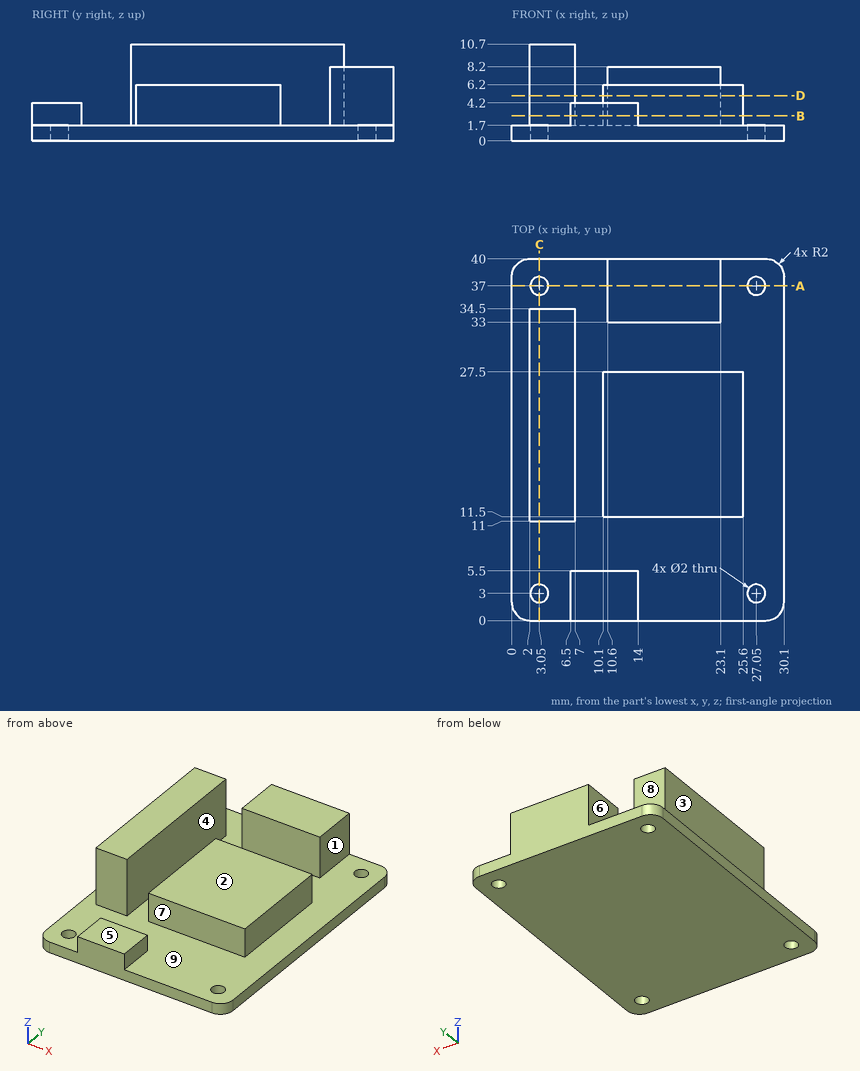
Geometry: see drawing. Coordinates: mm, zero at the bounding-box minimum. A direction names the side the tool comes from. Round coordinates to 2 decimals unless told otherwise and drop trailing zeros. Write each loop counter-clockwise with the first axis right and the second up, starting at its lowest first coordinate (ties: lowest second). Pieces come first, ordered by that corner, then holes. Notation, with made-up numbers: M 4.5,52.5 L 39.5,52.5 A20 cw 39.5,66.5 Z; hole C 79,14.5 d6. An arc over 180 degrees is marked long. Answer as a JSON object with one key per item and string values. Group by question number.
(1) Ray query, line 1 (Y direction, x = 27.05, z = 0.9); line 2 (X direction, y = 37, z = 0.6); line 3 (Y direction, x = 23, z = 5.25). Return the intervals inside material, ascending. Write a range as [from, to].
(2) Section query A-A on y = 37. Output: boundary loops of the cut face in (x, z).
(3) Reachability of the marked faces 1, 2, 3, 4 and 5 from +Z, -Z, +X, -X, +Y, -Y: full face, straight path, thin tool, end or side. Return the list, or none.
(4) Section query B-B on z = 2.75. Output: boundary loops of the cut face in (x, y).
(5) First-contact query: pin 1 (6 mm diameter, centred on x = 8.5, y = 2.5, fed in from +Z); pin 2 (6 mm diameter, centred on y = 10, z = 7, fed in from +X); pin 3 (1.9 mm diameter, centred on x = 17.5, z = 5.5, fed in from -Y); pin 4 (1.2 mm diameter, centred on x = 27.05, y = 37, fed in from -Z). Flat tips, straight axial feed; report the tip coordinate or a pass-through.
(6) Mould query, pull axis Y, two halves, no side actions, for the marked faces 6, 7, 8 and 9. Classes: +Y half, -Y half, draft (parallel to the pull), parting line (faces both ways), or undercut.
(7) Section query D-D on z = 5. Output: boundary loops of the cut face in (x, y), then the cut area to 3 significant figures.
(8) Section query C-C on x = 3.05. Output: boundary loops of the cut face in (y, z), then the cut area to 3 significant figures.
Computed values:
{
 "1": {"line 1": "[0, 2], [4, 36], [38, 40]", "line 2": "[0, 2.05], [4.05, 26.05], [28.05, 30.1]", "line 3": "[11.5, 27.5], [33, 40]"},
 "2": {"outline": "M 0,0 L 2.05,0 L 2.05,1.7 L 0,1.7 Z; M 4.05,0 L 26.05,0 L 26.05,1.7 L 23.1,1.7 L 23.1,8.2 L 10.6,8.2 L 10.6,1.7 L 4.05,1.7 Z; M 28.05,0 L 30.1,0 L 30.1,1.7 L 28.05,1.7 Z"},
 "3": {"face 1": "+Z, +X, +Y", "face 2": "+Z, +X, -Y", "face 3": "+Z, -X, +Y, -Y", "face 4": "+Z, +Y", "face 5": "+Z, +X, -X, -Y"},
 "4": {"outline": "M 2,11 L 7,11 L 7,34.5 L 2,34.5 Z; M 6.5,0 L 14,0 L 14,5.5 L 6.5,5.5 Z; M 10.1,11.5 L 25.6,11.5 L 25.6,27.5 L 10.1,27.5 Z; M 10.6,33 L 23.1,33 L 23.1,40 L 10.6,40 Z"},
 "5": {"pin 1": "z = 4.2", "pin 2": "x = 25.6", "pin 3": "y = 11.5", "pin 4": "through"},
 "6": {"face 6": "draft", "face 7": "undercut", "face 8": "+Y half", "face 9": "undercut"},
 "7": {"outline": "M 2,11 L 7,11 L 7,34.5 L 2,34.5 Z; M 10.1,11.5 L 25.6,11.5 L 25.6,27.5 L 10.1,27.5 Z; M 10.6,33 L 23.1,33 L 23.1,40 L 10.6,40 Z", "area": "453 mm^2"},
 "8": {"outline": "M 0,0 L 2,0 L 2,1.7 L 0,1.7 Z; M 4,0 L 36,0 L 36,1.7 L 34.5,1.7 L 34.5,10.7 L 11,10.7 L 11,1.7 L 4,1.7 Z; M 38,0 L 40,0 L 40,1.7 L 38,1.7 Z", "area": "273 mm^2"}
}
